For this review, take the finished solid that the model builds, in its own axes (mm). A direction names the side the tool comes from. Round coordinates to 2 decimals unless told otherwise and drop trailing zeros. Loops run counter-clockwise (first coordinate to the right, second up) from the corner with the lowest first, then second, coordinate; pieces in that order, holes last.
1. Tool access review of faces 4 (the cylindrical face through (5.354, -3.414, 42.113)), 5 (the flat face through (0, 6.35, 15)), 6 (the flat face through (-5.525, 3.131, 15.415)): name each direction out of +Z, -Z, +X, -X, +Y, -Y from which nothing blocks a thin tool from reaching the whole face with its end or side.
2. Consider section B-B on x = -0.75. State the section outline as (y, z) points, then the cut area to 3 significant figures.
3. Draft analysis for pull direction Z (two halves, no side actions). For faces 1 (the flat face through (0, 0, -45.244)), 2 (the flat face through (7, 0, 38.894)), 3 (the flat face through (-5.474, -3.219, 15.415)), state which applies: released by +Z, released by -Z, zero draft, split by the parting line, or undercut.
4. To check wall thickness, follow line 1 along Z through (x, y) = (2, -6.75); line 2 along Y through (x, z) = (5.5, 17); line 3 along Z through (x, y) = (-3, -6). State the ranges of each line that lie inside material, in increasing order.
5. Consider section A-A on z = 28.5. State the section outline as (x, y) points, then the cut area to 3 significant figures.
6. Clearance check with flat-ended pins moving along their axes: pin 1 Ø0.5 at (x, y) = (-6.5, 1.5) entering from +Z; pin 2 Ø3.5 at (x, z) = (0.5, 23) entering from +Y; pin 3 Ø1.5 at (y, z) = (4, -26.5) entering from -X. State where each tip first meets the part, or that it passes through.
7. Consider section D-D on z = -30. State the section outline as (x, y) points (1 decimal), then the cut area to 3 significant figures.
8. Consider section C-C on y = -5. State the section outline as (x, z) points, then the cut area to 3 significant figures.
Autodesk Inventor part; units mm, degrees
ref_plane "YZ Plane" through (0, 0, 0) normal (1, 0, 0) x (0, 1, 0)
ref_plane "XZ Plane" through (0, 0, 0) normal (0, 1, 0) x (-1, 0, 0)
ref_plane "XY Plane" through (0, 0, 0) normal (0, 0, 1) x (1, 0, 0)
sketch "Sketch1" plane through (0, 0, 0) normal (0, 0, 1) x (1, 0, 0)
  circle A0 centre (0, 0) radius 7.9375
  dimension "d0" = 15.875
extrude "Extrusion1" add sketch "Sketch1" along normal mid plane 90.4875
sketch "Sketch2" plane through (0, 0, 45.2437) normal (0, 0, 1) x (1, 0, 0)
  line L0 (-3.6662, 6.35) -> (3.6662, 6.35)
  line L1 (3.6662, 6.35) -> (7.3323, 0)
  line L2 (7.3323, 0) -> (3.6662, -6.35)
  line L3 (3.6662, -6.35) -> (-3.6662, -6.35)
  line L4 (-3.6662, -6.35) -> (-7.3323, 0)
  line L5 (-7.3323, 0) -> (-3.6662, 6.35)
  circle A0 centre (0, 0) radius 7.9375
  point P0 (0, -6.35)
  point P1 (0, 6.35)
  dimension "d3" = 12.7
extrude "Extrusion2" cut sketch "Sketch2" against normal blind 53.975
sketch "Sketch3" plane through (0, 0, 45.2437) normal (0, 0, 1) x (1, 0, 0)
  circle A0 centre (0, 0) radius 6.35
  circle A1 centre (0, 0) radius 7.9375
  line L0 (3.6662, 6.35) -> (-3.6662, 6.35)
  line L1 (7.3323, 0) -> (3.6662, 6.35)
  line L2 (3.6662, -6.35) -> (7.3323, 0)
  line L3 (-3.6662, -6.35) -> (3.6662, -6.35)
  line L4 (-7.3323, 0) -> (-3.6662, -6.35)
  line L5 (-3.6662, 6.35) -> (-7.3323, 0)
  point P0 (-5.4993, 3.175)
  point P1 (0, 6.35)
  point P2 (-5.4993, -3.175)
  point P3 (0, -6.35)
  point P4 (5.4993, -3.175)
  point P5 (5.4993, 3.175)
  dimension "d6" = 12.7
extrude "Extrusion3" cut sketch "Sketch3" against normal blind 6.35 contours A0 L1 L2 | A0 L0 L1 | L2 L3 A0 | A0 L5 L0 | L3 L4 A0 | A0 L4 L5
properties part number "EL2-C-007" material "Aluminum 6061"
Resolved:
1. face 4: +Z
1. face 5: +Z, +X, -X, +Y
1. face 6: +Z, -X, +Y
2. outline: (-7.9, -45.24) - (7.9, -45.24) - (7.9, -8.73) - (6.35, -8.73) - (6.35, 38.89) - (6.31, 38.89) - (6.31, 45.24) - (-6.31, 45.24) - (-6.31, 38.89) - (-6.35, 38.89) - (-6.35, -8.73) - (-7.9, -8.73) - close
2. area: 1,260 mm2
3. face 1: released by -Z
3. face 2: released by +Z
3. face 3: zero draft
4. line 1: z = -45.24 to -8.73
4. line 2: y = -3.17 to 3.17
4. line 3: z = -45.24 to 38.89
5. outline: (-7.33, 0) - (-3.67, -6.35) - (3.67, -6.35) - (7.33, 0) - (3.67, 6.35) - (-3.67, 6.35) - close
5. area: 140 mm2
6. pin 1: stops at z = 38.89
6. pin 2: stops at y = 6.35
6. pin 3: stops at x = -7.24
7. outline: circle Ø15.9 at (0, 0)
7. area: 198 mm2
8. outline: (-6.16, -45.24) - (6.16, -45.24) - (6.16, -8.73) - (4.45, -8.73) - (4.45, 38.89) - (3.91, 38.89) - (3.91, 45.24) - (-3.91, 45.24) - (-3.91, 38.89) - (-4.45, 38.89) - (-4.45, -8.73) - (-6.16, -8.73) - close
8. area: 923 mm2
